Geometry: final body of the model. Coordinates: model frame, mm. Give positions to 0.01 mm unless a question says otherwise; leave off trailing zeros. Order: outer loops, then holes, each group sorted by start corner. A loop starts at its lowest first (then second) coordinate and runs counter-clockwise, first axis right, second up. Notation, with made-up numbers: (41, 63.25) -> (45, 63.25) arc R32 ccw to (45, 93.25) -> close; hole circle Ø9 at (62.25, 86.25). An arc over 180 degrees is marked (long way). One line per question, with ' | ' between items. Start each with the question number.
(1) First-contact query: pin 1 Ø2.5 at (y, z) = (0, 18.26) entering from +X. Flat tip, straight axial feed; report the tip coordinate or a pass-through.
(2) Ray query, L1, parallel to X at y = -1.7, z = 28; L2, parallel to Y at x = -2, z = 5.5; L3, parallel to Y at x = -0.4, z = 63.5. Return the intervals inside material, ascending.
(3) Section A-A (z = 31.5). Return loops of the section in (x, y), then the cut area to 3 significant figures.
(4) Section B-B (x = 0). State how many separate pieces and enclosed holes the cut face has, then the cut area to 3 significant figures.
Autodesk Inventor part; units mm, degrees
ref_plane "YZ Plane" through (0, 0, 0) normal (1, 0, 0) x (0, 1, 0)
ref_plane "XZ Plane" through (0, 0, 0) normal (0, 1, 0) x (-1, 0, 0)
ref_plane "XY Plane" through (0, 0, 0) normal (0, 0, 1) x (1, 0, 0)
sketch "Sketch1" plane through (0, 0, 0) normal (0, 0, 1) x (1, 0, 0)
  line L0 (-2.3812, -2.3813) -> (2.3813, -2.3813)
  line L1 (2.3813, -2.3813) -> (2.3812, 2.3812)
  line L2 (2.3812, 2.3812) -> (-2.3813, 2.3812)
  line L3 (-2.3813, 2.3812) -> (-2.3812, -2.3813)
  line L4 (-2.3812, -2.3813) -> (2.3812, 2.3812) construction
  line L5 (2.3813, -2.3813) -> (-2.3813, 2.3812) construction
  point P0 (0, 0)
  dimension "d0" = 4.7625
  dimension "d1" = 4.7625
extrude "Extrusion1" add sketch "Sketch1" along normal blind 96.8375
sketch "Sketch2" plane through (-2.3813, 2.3812, 0) normal (0, 1, 0) x (1, 0, 0)
  line L0 (2.3813, 0) -> (2.3813, -96.8375) construction
  line L1 (4.7625, -96.8375) -> (0, -96.8375)
  circle A0 centre (2.3813, -2.3813) radius 1.4732
  circle A1 centre (2.3813, -8.7313) radius 1.4732
  circle A2 centre (2.3813, -15.0813) radius 1.4732
  circle A3 centre (2.3813, -21.4313) radius 1.4732
  circle A4 centre (2.3813, -26.1938) radius 1.4493 construction
  line L2 (4.7625, 0) -> (0, 0)
  circle A5 centre (2.3813, -27.7812) radius 1.4732
  circle A6 centre (2.3813, -34.1313) radius 1.4732
  circle A7 centre (2.3813, -40.4812) radius 1.4732
  circle A8 centre (2.3813, -46.8313) radius 1.4732
  circle A9 centre (2.3813, -53.1813) radius 1.4732
  circle A10 centre (2.3813, -59.5312) radius 1.4732
  circle A11 centre (2.3813, -65.8812) radius 1.4732
  circle A12 centre (2.3813, -72.2313) radius 1.4732
  circle A13 centre (2.3813, -78.5812) radius 1.4732
  circle A14 centre (2.3813, -84.9313) radius 1.4732
  circle A15 centre (2.3813, -91.2812) radius 1.4732
  dimension "d4" = 2.9464
  dimension "d7" = 6.35
  dimension "d12" = 4.7625
  dimension "d13" = 2.3813
extrude "Extrusion2" cut sketch "Sketch2" against normal through all
sketch "Sketch3" plane through (2.3813, -2.3813, 0) normal (1, 0, 0) x (0, 0, -1)
  line L0 (0, 2.3813) -> (-96.8375, 2.3813) construction
  line L1 (-96.8375, 0) -> (-96.8375, 4.7625)
  circle A0 centre (-94.4562, 2.3813) radius 1.4732
  circle A1 centre (-88.1063, 2.3813) radius 1.4732
  circle A2 centre (-81.7562, 2.3813) radius 1.4732
  circle A3 centre (-75.4062, 2.3813) radius 1.4732
  circle A4 centre (-69.0562, 2.3813) radius 1.4732
  circle A5 centre (-62.7062, 2.3813) radius 1.4732
  circle A6 centre (-56.3562, 2.3813) radius 1.4732
  circle A7 centre (-50.0062, 2.3813) radius 1.4732
  circle A8 centre (-43.6562, 2.3813) radius 1.4732
  circle A9 centre (-37.3062, 2.3813) radius 1.4732
  circle A10 centre (-30.9563, 2.3813) radius 1.4732
  circle A11 centre (-24.6062, 2.3813) radius 1.4732
  circle A12 centre (-18.2562, 2.3813) radius 1.4732
  circle A13 centre (-11.9062, 2.3813) radius 1.4732
  circle A14 centre (-5.5562, 2.3813) radius 1.4732
  dimension "d16" = 2.9464
  dimension "d17" = 2.3813
  dimension "d20" = 6.35
extrude "Extrusion3" cut sketch "Sketch3" against normal through all
chamfer "Chamfer1" distance 0.1 angle 45 4 edges at (-2.3813, 2.3812, 48.4188) (2.3812, 2.3812, 48.4188) (2.3813, -2.3813, 48.4188) (-2.3812, -2.3813, 48.4188)
equation "\"d1\" = d0"
properties part number "Nut Strip" material "Aluminum 6061"
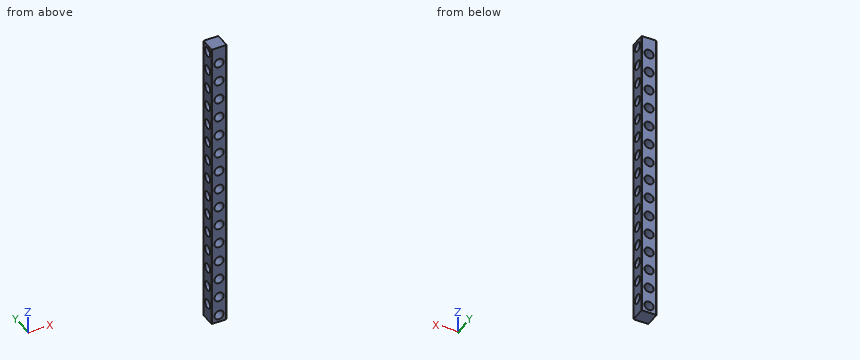
Response:
1) pin 1: passes through
2) L1: x = -2.38 to -1.46, 1.46 to 2.38 | L2: y = -2.38 to -1.47, 1.47 to 2.38 | L3: y = -2.38 to -1.24, 1.24 to 2.38
3) outline: (-2.38, -2.28) -> (-2.28, -2.38) -> (2.28, -2.38) -> (2.38, -2.28) -> (2.38, -1.37) -> (-2.38, -1.37) -> close; (-2.38, 1.37) -> (2.38, 1.37) -> (2.38, 2.28) -> (2.28, 2.38) -> (-2.28, 2.38) -> (-2.38, 2.28) -> close | area: 9.62 mm^2
4) separate pieces: 16 | enclosed holes: 15 | area: 148 mm^2
